Could you check a few things on this drawing? It's one solid part, dimensions in mm from its lowest x, y, z. A direction names the side the tool comes from. Coordinates: 2 decimals unless noted, no trailing zeros. Loops run counter-clockwise (first coordinate to the right, second up) from the corner with the lowest first, then second, coordinate; pieces in that order, holes last. Notation, with made-up numbers: (80.5, -34) -> (123.5, -34) arc R26 cw to (123.5, 2) -> close; hole circle Ø4 at (20.25, 21.5). An arc over 180 degrees is marked (long way). One line per question, with ' | ' between items.
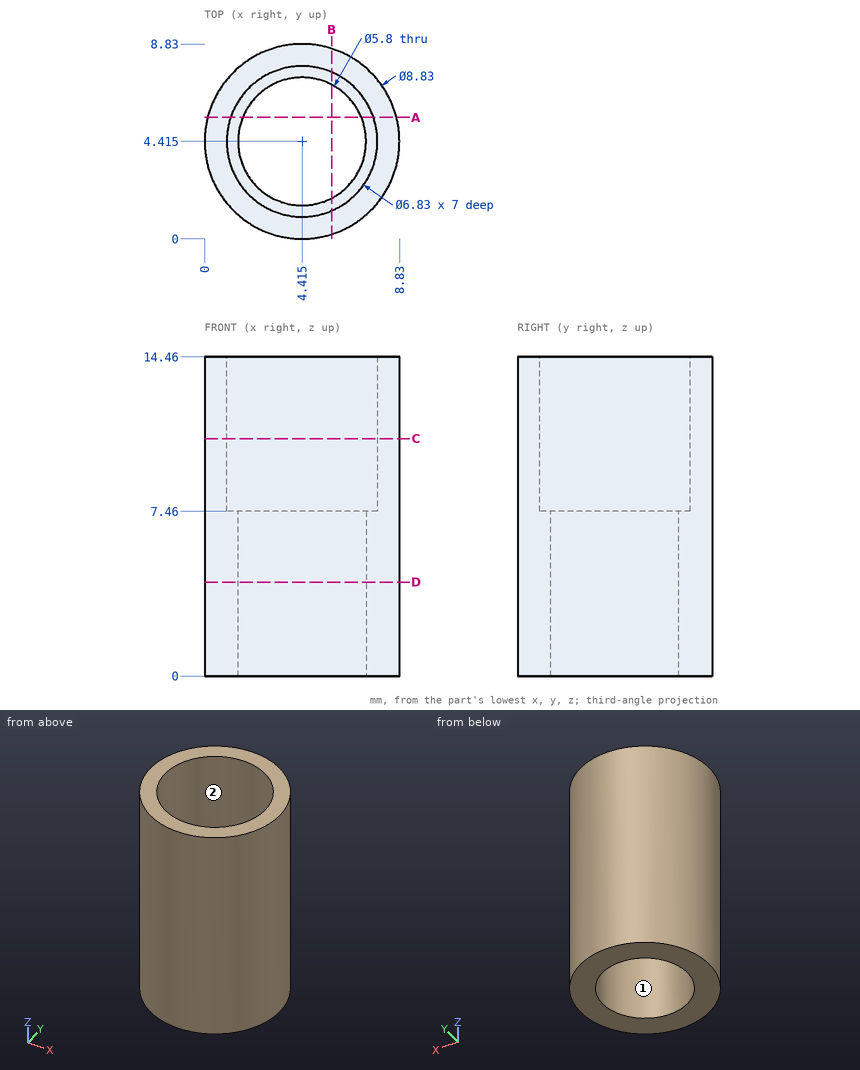
1) On a 3-axis mill with a long thin cutter (end or side, diameter ignored), from which of +Z, -Z, +X, -X, +Y, -Y can I reach the whole of each face in a straight line? I mean the marked faces 1 and 2. Say none if no direction works.
Data:
face 1: +Z, -Z | face 2: +Z
2) If we section it at C-C on z = 10.75: Please give me the cut outline in (x, y) (3 decimals), and give its area (3 significant figures).
Data:
outline: circle Ø8.83 at (4.415, 4.415); hole circle Ø6.83 at (4.415, 4.415) | area: 24.6 mm²
3) I need wall thicknesses on line 1 along Y through (x, z) = (4.5, 8.25); line 2 along Z through (x, y) = (2.5, 6.75); line 3 along X through (y, z) = (3.25, 11.75). Which ranges of each line are inside material? Lowest first, please. Write a range as from..to.
Data:
line 1: 0..1, 7.83..8.83 | line 2: 0..7.46 | line 3: 0.16..1.2, 7.63..8.67
4) If we section it at B-B on x = 5.75: Please give me the cut outline in (y, z), and give its area (3 significant figures).
Data:
outline: (0.21, 0) -> (1.84, 0) -> (1.84, 7.46) -> (1.27, 7.46) -> (1.27, 14.46) -> (0.21, 14.46) -> close; (6.99, 0) -> (8.62, 0) -> (8.62, 14.46) -> (7.56, 14.46) -> (7.56, 7.46) -> (6.99, 7.46) -> close | area: 39.3 mm²
5) If we section it at A-A on y = 5.5: Please give me the cut outline in (x, z), and give its area (3 significant figures).
Data:
outline: (0.14, 0) -> (1.73, 0) -> (1.73, 7.46) -> (1.18, 7.46) -> (1.18, 14.46) -> (0.14, 14.46) -> close; (7.1, 0) -> (8.69, 0) -> (8.69, 14.46) -> (7.65, 14.46) -> (7.65, 7.46) -> (7.1, 7.46) -> close | area: 38.3 mm²
6) If we section it at D-D on z = 4.25: Please give me the cut outline in (x, y) (3 decimals), and give its area (3 significant figures).
Data:
outline: circle Ø8.83 at (4.415, 4.415); hole circle Ø5.8 at (4.415, 4.415) | area: 34.8 mm²
7) I'm going to push flat-ended pins straight in: pin 1 Ø2 at (y, z) = (3, 2) entering from +X; pin 2 Ø2 at (x, z) = (2.5, 2) entering from -Y. Where does each tip first touch, or does it pass through?
Data:
pin 1: x = 8.81 | pin 2: y = 0.1
